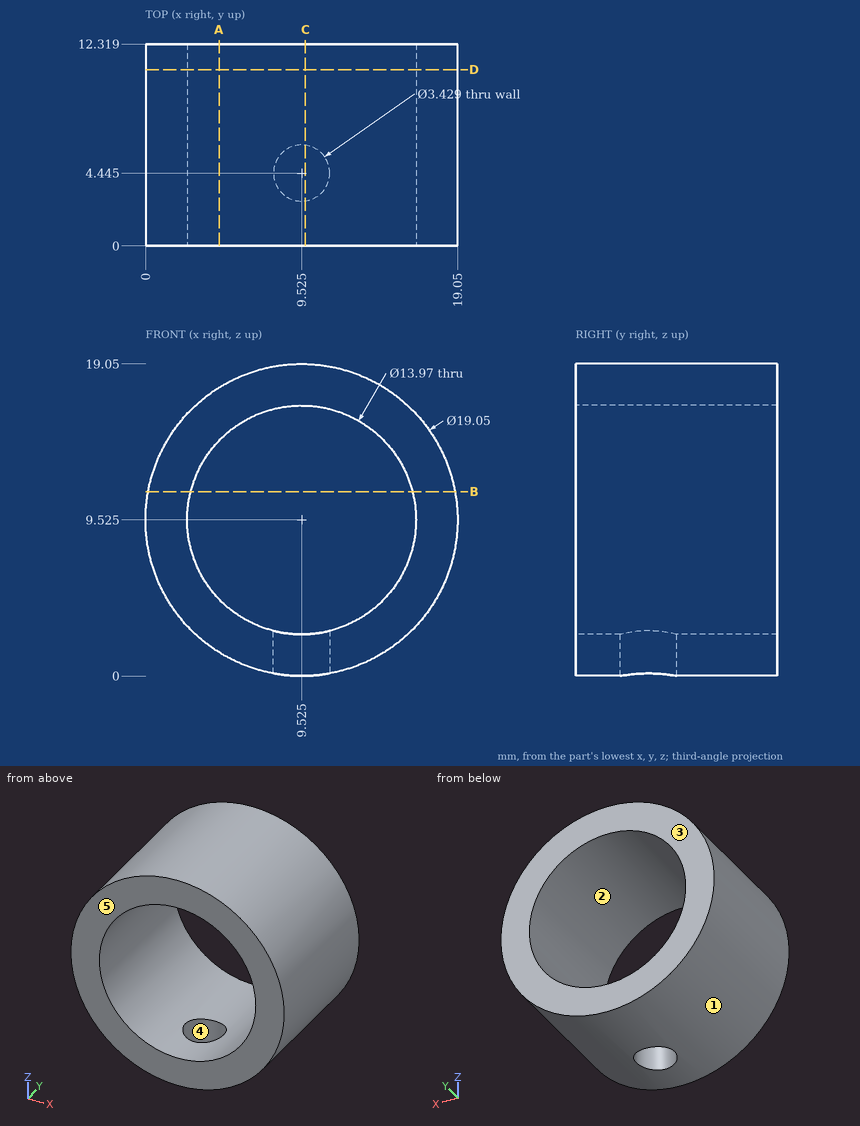
Design review of the part shown in the three views and the two pictorial views. Dimensions are in mm from the part's minimum x, y and z. A direction names the side the tool comes from. Give positions to 0.01 mm unless a question says otherwise; leave off trailing zeros. Loops run counter-clockwise (first coordinate to the right, second up) from the corner with the lowest first, then second, coordinate; pieces in that order, holes last. Notation, with made-up numbers: (-2.75, 26.25) -> (44.25, 26.25) arc R20 cw to (44.25, 45.25) -> close; hole circle Ø5 at (-3, 24.5). An arc over 180 degrees is marked (long way). One line per item, written item: value.
Q1. Machinability: for the marked faces 4 and 5, which of the approach directions +Z, -Z, +X, -X, +Y, -Y give a long, thin tool a straight path to every point of the face, cutting with its end or side? Answer none if there is none.
Numbers:
face 4: -Z
face 5: +Z, -Z, +X, -X, -Y
Q2. Draft analysis for pull direction X (two halves, no side actions). For the marked faces 1, 2 and 3, state which applies: pulls with the +X half, pulls with the -X half, needs draft (parallel to the pull), parting line crosses it, or undercut.
Numbers:
face 1: parting line crosses it
face 2: undercut
face 3: needs draft
Q3. We need section A-A on x = 4.5. Give the boundary of the cut face in (y, z).
Numbers:
outline: (0, 1.43) -> (12.32, 1.43) -> (12.32, 4.67) -> (0, 4.67) -> close; (0, 14.38) -> (12.32, 14.38) -> (12.32, 17.62) -> (0, 17.62) -> close
Q4. We need section B-B on z = 11.25. Give the boundary of the cut face in (x, y), and give its area (3 significant figures).
Numbers:
outline: (0.16, 0) -> (2.76, 0) -> (2.76, 12.32) -> (0.16, 12.32) -> close; (16.29, 0) -> (18.89, 0) -> (18.89, 12.32) -> (16.29, 12.32) -> close
area: 64.0 mm^2
Q5. We need section C-C on x = 9.75. Give the boundary of the cut face in (y, z), and give its area (3 significant figures).
Numbers:
outline: (0, 0) -> (2.75, 0) -> (2.75, 2.54) -> (0, 2.54) -> close; (0, 16.51) -> (12.32, 16.51) -> (12.32, 19.05) -> (0, 19.05) -> close; (6.14, 0) -> (12.32, 0) -> (12.32, 2.54) -> (6.14, 2.54) -> close
area: 54.0 mm^2
Q6. For L1, parallel to Z at x = 9.5, y = 11.25; L2, parallel to X at y = 0.5, z = 5.5, list the stretches that pass through material, from the lowest coordinate up.
Numbers:
L1: z = 0 to 2.54, 16.51 to 19.05
L2: x = 0.89 to 3.82, 15.23 to 18.16
Q7. We need section D-D on y = 10.75. Give the boundary of the cut face in (x, z) (3 decimals).
Numbers:
outline: circle Ø19.05 at (9.525, 9.525); hole circle Ø13.97 at (9.525, 9.525)
Q8. For pin 1 Ø5 at (x, y) = (11.5, 5) entering from -Z; pin 2 Ø4 at (y, z) = (9.5, 3) entering from +X; pin 3 Ø4 at (y, z) = (6.5, 6) entering from -X; pin 4 Ø11 at (x, z) = (9.525, 9.525) entering from -Y, all flat-tipped, find the tip position at first contact; note any pin that passes through.
Numbers:
pin 1: stops at z = 0
pin 2: stops at x = 17.91
pin 3: stops at x = 0.12
pin 4: passes through
